Design review of the part built by this model. Coordinates are the model's own, in mm. A direction names the side the tool comes from. Coordinates: 2 decimals unless noted, no trailing zeros. Write each loop counter-clockwise with the first axis right and the second up, starting at its lowest first coordinate (ties: lowest second). Pieces come first, ordered by that corner, then holes. Notation, with made-up numbers: M 45.5,-36 L 68.5,-36 A36 cw 68.5,-2 Z; hole C 17,89 d10. An arc over 180 degrees is marked long. Write each question's results on one line, items separated by ' | '. Start each with the question number.
Autodesk Inventor part; units mm, degrees
ref_plane "YZ Plane" through (0, 0, 0) normal (1, 0, 0) x (0, 1, 0)
ref_plane "XZ Plane" through (0, 0, 0) normal (0, 1, 0) x (-1, 0, 0)
ref_plane "XY Plane" through (0, 0, 0) normal (0, 0, 1) x (1, 0, 0)
ref_plane "Arbeitsebene1" through (-7.5, 0, 0) normal (0, 0, 1) x (1, 0, 0)
sketch "Skizze1" plane through (-7.5, 0, 0) normal (0, 0, 1) x (1, 0, 0)
  line L0 (-71.1, -93.5) -> (-71.1, 90.5)
  line L1 (62.9, -94.5) -> (-70.1, -94.5)
  line L2 (63.9, 90.5) -> (63.9, -93.5)
  line L3 (-70.1, 91.5) -> (62.9, 91.5)
  line L4 (23.9, -70.5) -> (-66.1, -70.5)
  line L5 (-66.1, -70.5) -> (-66.1, 73.5)
  line L6 (-66.1, 73.5) -> (23.9, 73.5)
  line L7 (23.9, 73.5) -> (23.9, -70.5)
  line L8 (8.9, -87.5) -> (-1.1, -87.5)
  line L9 (-1.1, -87.5) -> (-1.1, -77.5)
  line L10 (-1.1, -77.5) -> (8.9, -77.5)
  line L11 (8.9, -77.5) -> (8.9, -73.5)
  line L12 (8.9, -73.5) -> (26.9, -73.5)
  line L13 (26.9, -73.5) -> (26.9, -56.5)
  line L14 (26.9, -56.5) -> (60.9, -56.5)
  line L15 (60.9, -56.5) -> (60.9, -91.5)
  line L16 (60.9, -91.5) -> (8.9, -91.5)
  line L17 (8.9, -91.5) -> (8.9, -87.5)
  line L18 (-0.95, -77.65) -> (-0.95, -87.35)
  line L19 (-0.95, -87.35) -> (9.05, -87.35)
  line L20 (9.05, -87.35) -> (9.05, -91.35)
  line L21 (9.05, -91.35) -> (60.75, -91.35)
  line L22 (60.75, -91.35) -> (60.75, -56.65)
  line L23 (60.75, -56.65) -> (27.05, -56.65)
  line L24 (27.05, -56.65) -> (27.05, -73.65)
  line L25 (27.05, -73.65) -> (9.05, -73.65)
  line L26 (9.05, -73.65) -> (9.05, -77.65)
  line L27 (9.05, -77.65) -> (-0.95, -77.65)
  line L28 (63.9, -93.5) -> (62.9, -94.5)
  line L29 (62.9, 91.5) -> (63.9, 90.5)
  line L30 (-71.1, 90.5) -> (-70.1, 91.5)
  line L31 (-70.1, -94.5) -> (-71.1, -93.5)
  circle A0 centre (43.9, -1.5) radius 7.55
  circle A1 centre (-61.1, -85.5) radius 7.55
  circle A2 centre (-61.1, 82.5) radius 7.55
  point P0 (7.5, 0)
  dimension "d0" = 0.15
extrude "Extrusion1" add sketch "Skizze1" against normal blind 3.6 contours L27 L26 L25 L24 L23 L22 L21 L20 L19 L18
sketch "Skizze2" plane through (-7.5, 0, 0) normal (0, 0, 1) x (1, 0, 0)
  circle A0 centre (3.9, -82.5) radius 2
  point P0 (7.5, 0)
hole "Bohrung1" at (-3.6, -82.5, 0) direction (0, 0, -1) diameter 3.4 depth 8 countersink diameter 7.5 countersink angle 90
sketch "Skizze3" plane through (53.25, -91.35, 0) normal (1, 0, 0) x (0, 0, -1)
  line L0 (2, 27.35) -> (2, 7.35)
  line L1 (2, 7.35) -> (3.6, 7.35)
  line L2 (3.6, 7.35) -> (3.6, 27.35)
  line L3 (3.6, 27.35) -> (2, 27.35)
  line L4 (2, 27.35) -> (2, 7.35)
  point P0 (0, 91.35)
  point P1 (3.6, 34.7)
extrude "Extrusion2" add sketch "Skizze3" along normal blind 2
chamfer "Fasen1" distance 0.5 angle 45 7 edges at (-8.45, -87.35, -1.8) (-8.45, -77.65, -1.8) (1.55, -73.65, -1.8) (1.55, -91.35, -1.8) (19.55, -56.65, -1.8) (53.25, -56.65, -1.8) (53.25, -91.35, -1.8)
chamfer "Fasen2" distance 0.5 angle 45 3 edges at (55.25, -84, -2.8) (55.25, -64, -2.8) (55.25, -74, -2)
properties part number "Kameraturm_Abdeckung_Unten"
Item 1: Draft analysis for pull direction X (two halves, no side actions). For faces 1 (the flat face through (1.55, -76, -2)), 2 (the cylindrical face through (-3.67, -80.8, -2.84)), 3 (the flat face through (27, -91.35, -2)), 4 (the flat face through (55.25, -74, -3)), state which applies: released by +X, released by -X, zero draft, split by the parting line, or undercut.
Item 2: We need section D-D on x = 14. State the section outline as (y, z) points, then the cut area to 3 significant figures.
Item 3: We need section A-A on y = -82.5. State the section outline as (x, z) points, then the cut area to 3 significant figures.
Item 4: Insertion check: pin 1 Ø1.1 at (x, z) = (-3.5, -1.5) entering from +Y; pin 2 Ø0.8 at (x, z) = (54.5, -3) entering from -Y; pin 3 Ø0.8 at (x, y) = (54.5, -73.5) entering from +Z. Each pin has a flat end and moves straight along its axis. Give the tip position at first contact, or say it passes through.
Item 5: We need section C-C on z = -1.4. State the section outline as (x, y) points, then the cut area to 3 significant figures.
Item 6: For faces 5 (the flat face through (54, -84, -3)), 6 (the flat face through (19.55, -65, -2)), 7 (the flat face through (54, -64, -3)), 8 (the flat face through (1.55, -89, -2)), list the 3-axis set-ups (+Z, -Z, +X, -X, +Y, -Y) from which the entire face can be reached by the end or side of a thin tool; tool diameter is ignored.
Item 7: We need section B-B on x = -3.6. State the section outline as (y, z) points, then the cut area to 3 significant figures.
Item 8: Wall thickness on L1, parallel to X at y = -82.5, z = -2.5; L2, parallel to Y at x = -3.6, z = -2.65; L3, parallel to Y at x = 1.5, z = -1.3: over which ranges is each line inside the solid? List them lowest first.
Answer:
1) face 1: released by -X | face 2: undercut | face 3: zero draft | face 4: released by +X
2) outline: M -91.35,-3.6 L -73.65,-3.6 L -73.65,0 L -91.35,0 Z | area: 63.7 mm^2
3) outline: M -8.45,-3.6 L -5.3,-3.6 L -5.3,-2.05 L -7.35,0 L -8.45,0 Z; M -1.9,-3.6 L 55.25,-3.6 L 55.25,-2.5 L 54.75,-2 L 53.25,-2 L 53.25,0 L 0.15,0 L -1.9,-2.05 Z | area: 209 mm^2
4) pin 1: stops at y = -77.65 | pin 2: stops at y = -84 | pin 3: stops at z = -2
5) outline: M -8.45,-86.85 L -7.95,-87.35 L 1.55,-87.35 L 1.55,-90.85 L 2.05,-91.35 L 52.75,-91.35 L 53.25,-90.85 L 53.25,-57.15 L 52.75,-56.65 L 20.05,-56.65 L 19.55,-57.15 L 19.55,-73.65 L 2.05,-73.65 L 1.55,-74.15 L 1.55,-77.65 L -7.95,-77.65 L -8.45,-78.15 Z; hole C -3.6,-82.5 d4.7 | area: 1,570 mm^2
6) face 5: +Z, -Z, +X, -Y | face 6: +Z, -Z, -X, +Y | face 7: +Z, -Z, +X, +Y | face 8: +Z, -Z, -X, -Y
7) outline: M -87.35,-3.6 L -84.2,-3.6 L -84.2,-2.05 L -86.25,0 L -87.35,0 Z; M -80.8,-3.6 L -77.65,-3.6 L -77.65,0 L -78.75,0 L -80.8,-2.05 Z | area: 18.5 mm^2
8) L1: x = -8.45 to -5.3, -1.9 to 55.25 | L2: y = -87.35 to -84.2, -80.8 to -77.65 | L3: y = -87.35 to -77.65
